Can you work these out from the model? Positions are in its coordinate system, mm. A direction names the side the tool comes from. Coordinates: 2 decimals unless noted, no trailing zeros. Loops run counter-clockwise (first coordinate to the right, second up) from the corner with the lowest first, then second, coordinate; pieces in that order, holes last. Notation, with made-up numbers: (-25.5, 53.5) -> (18.5, 53.5) arc R25 ccw to (18.5, 87.5) -> close; hole circle Ø7 at (56.5, -5). An arc over 180 degrees is marked (long way). Put each result on its own line as item: value. Start each with the question number.
Item 1: Will these pins go through, and if not, where does the flat tip stop? P1, Ø0.6, axis at x = -6.5, y = -17.5, coming from the -Z side; P2, Ø6, axis at x = 0, z = 0, coming from the -Y side; P3, Ø8, axis at x = -0.5, y = -21.5, coming from the +Z side.
Item 2: If we section it at A-A on z = 0: Please give me the cut outline in (x, y).
Item 3: If we section it at C-C on y = -17.5: Please give me the cut outline in (x, z).
Item 4: We'd pull the mould along Y, two halves only. Please class faces 1 (the flat face through (-7, -15, 1.4)), 2 (the flat face through (5.85, 6.52, -5.91)), 3 (the flat face through (-6, 2, -7)), 4 (the cylindrical face through (-6.9, -21.4, 0)): pulls with the +Y half, pulls with the -Y half, needs draft (parallel to the pull), parting line crosses it, or undercut.
Item 5: If we section it at D-D on y = -26.5: Please give me the cut outline in (x, z), plus the area to 3 significant figures.
Item 6: For faces 5 (the flat face through (-6, 0, -6)), 6 (the flat face through (-8.5, 2, 0)), 7 (the flat face through (-7, -15, -1.4)), 8 (the flat face through (0, 2, 0)), which set-ups out of +Z, -Z, +X, -X, +Y, -Y let a thin tool reach every point of the face, with its end or its side?
Item 7: Please list where these lines run through material, in increasing order: L1, parallel to Y at x = -1.25, z = 5; L2, parallel to X at y = -21, z = 0; L3, parallel to Z at x = 4, y = -9. Write a range as from..to.
Item 8: If we section it at B-B on x = 0: Please give me the cut outline in (y, z).
```python
from build123d import *
from OCP.BRepFilletAPI import BRepFilletAPI_MakeChamfer

# Parameters (mm, degrees)
SKETCH1_W           = 17
SKETCH1_H           = 17
BOSS_EXTRUDE1_DEPTH = 8
SKETCH5_R           = 8
BOSS_EXTRUDE3_DEPTH = 30
SKETCH6_R           = 6
CUT_EXTRUDE5_DEPTH  = 30
CUT_EXTRUDE6_DEPTH  = 33.318725222
CHAMFER1_SIZE       = 4
SKETCH11_R          = 5
CUT_EXTRUDE7_DEPTH  = 6
CHAMFER2_SIZE       = 3
CHAMFER2_SIZE2      = 1.732050808


with BuildPart() as part:
    # Sketch1 → Boss-Extrude1 (new body)
    with BuildSketch(Plane(origin=(0, 0, 0), x_dir=(1, 0, 0), z_dir=(0, 1, 0))):
        Rectangle(SKETCH1_W, SKETCH1_H)
    extrude(amount=BOSS_EXTRUDE1_DEPTH)

    # Sketch5 → Boss-Extrude3 (add)
    with BuildSketch(Plane.XZ):
        with Locations(Location((0, 0, 0), (0, 0, 270))):
            Circle(SKETCH5_R)
    extrude(amount=BOSS_EXTRUDE3_DEPTH)

    # Sketch6 → Cut-Extrude5 (cut)
    with BuildSketch(Plane.XZ.offset(30)):
        with Locations(Location((0, 0, 0), (0, 0, 270))):
            Circle(SKETCH6_R)
    extrude(amount=-CUT_EXTRUDE5_DEPTH, mode=Mode.SUBTRACT)

    # Sketch8 → Cut-Extrude6 (cut, through all)
    with BuildSketch(Plane(origin=(0, 0, 0), x_dir=(0, 0, -1), z_dir=(1, 0, 0))):
        with BuildLine():
            Line((-1.4, -20), (-1.4, -10))
            ThreePointArc((-1.4, -10), (0, -8.6), (1.4, -10))
            Line((1.4, -10), (1.4, -20))
            ThreePointArc((1.4, -20), (0, -21.4), (-1.4, -20))
        make_face()
    extrude(amount=-CUT_EXTRUDE6_DEPTH, mode=Mode.SUBTRACT)

    # Chamfer1
    chamfer1_edges = [part.edges().sort_by_distance(p)[0] for p in [
        (8.5, 4, 8.5),
        (-8.5, 4, 8.5),
        (-8.5, 4, -8.5),
        (8.5, 4, -8.5),
    ]]
    chamfer(chamfer1_edges, length=CHAMFER1_SIZE)

    # Sketch11 → Cut-Extrude7 (cut)
    with BuildSketch(Plane(origin=(0, 8, 0), x_dir=(1, 0, 0), z_dir=(0, 1, 0))):
        with Locations(Location((0, 0, 0), (0, 0, 270))):
            Circle(SKETCH11_R)
    extrude(amount=-CUT_EXTRUDE7_DEPTH, mode=Mode.SUBTRACT)

    # Chamfer2: one chamfer whose edges measure the first distance from different faces: ONE call of the kernel's chamfer builder (chamfer() names one face for all edges)
    chamfer2_edges_1 = [part.edges().sort_by_distance(p)[0] for p in [
        (0, 8, 8.5),
    ]]
    chamfer2_side_1 = [part.faces().sort_by_distance(p)[0] for p in [
        (0, 4, 8.5),
    ]]
    chamfer2_edges_2 = [part.edges().sort_by_distance(p)[0] for p in [
        (-8.5, 8, 0),
    ]]
    chamfer2_side_2 = [part.faces().sort_by_distance(p)[0] for p in [
        (-8.5, 4, 0),
    ]]
    chamfer2_edges_3 = [part.edges().sort_by_distance(p)[0] for p in [
        (8.5, 8, 0),
    ]]
    chamfer2_side_3 = [part.faces().sort_by_distance(p)[0] for p in [
        (8.5, 4, 0),
    ]]
    chamfer2_edges_4 = [part.edges().sort_by_distance(p)[0] for p in [
        (0, 8, -8.5),
    ]]
    chamfer2_side_4 = [part.faces().sort_by_distance(p)[0] for p in [
        (0, 4, -8.5),
    ]]
    chamfer2_edges_5 = [part.edges().sort_by_distance(p)[0] for p in [
        (6.5, 8, -6.5),
    ]]
    chamfer2_side_5 = [part.faces().sort_by_distance(p)[0] for p in [
        (6.5, 4, -6.5),
    ]]
    chamfer2_edges_6 = [part.edges().sort_by_distance(p)[0] for p in [
        (-6.5, 8, -6.5),
    ]]
    chamfer2_side_6 = [part.faces().sort_by_distance(p)[0] for p in [
        (-6.5, 4, -6.5),
    ]]
    chamfer2_edges_7 = [part.edges().sort_by_distance(p)[0] for p in [
        (6.5, 8, 6.5),
    ]]
    chamfer2_side_7 = [part.faces().sort_by_distance(p)[0] for p in [
        (6.5, 4, 6.5),
    ]]
    chamfer2_edges_8 = [part.edges().sort_by_distance(p)[0] for p in [
        (-6.5, 8, 6.5),
    ]]
    chamfer2_side_8 = [part.faces().sort_by_distance(p)[0] for p in [
        (-6.5, 4, 6.5),
    ]]
    chamfer2 = BRepFilletAPI_MakeChamfer(part.part.solid().wrapped)
    for e in chamfer2_edges_1:
        chamfer2.Add(CHAMFER2_SIZE, CHAMFER2_SIZE2, e.wrapped, chamfer2_side_1[0].wrapped)  # the first distance lies on this face
    for e in chamfer2_edges_2:
        chamfer2.Add(CHAMFER2_SIZE, CHAMFER2_SIZE2, e.wrapped, chamfer2_side_2[0].wrapped)  # the first distance lies on this face
    for e in chamfer2_edges_3:
        chamfer2.Add(CHAMFER2_SIZE, CHAMFER2_SIZE2, e.wrapped, chamfer2_side_3[0].wrapped)  # the first distance lies on this face
    for e in chamfer2_edges_4:
        chamfer2.Add(CHAMFER2_SIZE, CHAMFER2_SIZE2, e.wrapped, chamfer2_side_4[0].wrapped)  # the first distance lies on this face
    for e in chamfer2_edges_5:
        chamfer2.Add(CHAMFER2_SIZE, CHAMFER2_SIZE2, e.wrapped, chamfer2_side_5[0].wrapped)  # the first distance lies on this face
    for e in chamfer2_edges_6:
        chamfer2.Add(CHAMFER2_SIZE, CHAMFER2_SIZE2, e.wrapped, chamfer2_side_6[0].wrapped)  # the first distance lies on this face
    for e in chamfer2_edges_7:
        chamfer2.Add(CHAMFER2_SIZE, CHAMFER2_SIZE2, e.wrapped, chamfer2_side_7[0].wrapped)  # the first distance lies on this face
    for e in chamfer2_edges_8:
        chamfer2.Add(CHAMFER2_SIZE, CHAMFER2_SIZE2, e.wrapped, chamfer2_side_8[0].wrapped)  # the first distance lies on this face
    add(Compound.cast(chamfer2.Shape()), mode=Mode.REPLACE)


solid = part.part
```
Solutions:
1. P1: z = -5.06
1. P2: y = 0
1. P3: z = 8
2. outline: (-8.5, 0) -> (-8, 0) -> (-8, -8.6) -> (-6, -8.6) -> (-6, 0) -> (6, 0) -> (6, -30) -> (8, -30) -> (8, 0) -> (8.5, 0) -> (8.5, 5) -> (6.77, 8) -> (5, 8) -> (5, 2) -> (-5, 2) -> (-5, 8) -> (-6.77, 8) -> (-8.5, 5) -> close; (-8, -30) -> (-6, -30) -> (-6, -21.4) -> (-8, -21.4) -> close
3. outline: (-7.88, -1.4) arc R8 ccw (long way) to (-7.88, 1.4) -> (-5.83, 1.4) arc R6 cw (long way) to (-5.83, -1.4) -> close
4. face 1: undercut
4. face 2: pulls with the +Y half
4. face 3: needs draft
4. face 4: undercut
5. outline: circle Ø16 at (0, 0); hole circle Ø12 at (0, 0)
5. area: 88.0 mm^2
6. face 5: -Y
6. face 6: +Z, -Z, -X, +Y, -Y
6. face 7: -X
6. face 8: +Y
7. L1: 0..8
7. L2: 6..8
7. L3: -6.93..-4.47, 4.47..6.93
8. outline: (-30, -8) -> (0, -8) -> (0, -8.5) -> (5, -8.5) -> (8, -6.77) -> (8, -5) -> (2, -5) -> (2, 5) -> (8, 5) -> (8, 6.77) -> (5, 8.5) -> (0, 8.5) -> (0, 8) -> (-30, 8) -> (-30, 6) -> (0, 6) -> (0, -6) -> (-30, -6) -> close
